Source: CAD feature listing. Evaluate the final solid. Frame: model axes, mm. A direction names the side the tool comes from. Give positions to 0.01 mm unless a question says otherwise; leave off trailing zeros. Write each loop counter-clockwise with the first axis right and the second up, starting at its lowest first coordinate (ties: lowest second). Pieces come first, ordered by that corner, then holes. Notation, with made-up numbers: (3.5, 86) -> (11.5, 86) arc R17 ccw to (11.5, 91) -> close; hole circle Ø7 at (-0.5, 46.25). An arc over 180 degrees is marked (long way). Use one line per item in the form item = value. Start each with the question number.
(1) Cut plane C-C, the plane z = 6.5. Count the separate pieces of the cut face and the enclosed holes in it, and give its area (3 significant figures).
(2) Material intervals for line 1 along Y through (x, z) = (13, 47); line 2 along Y through (x, z) = (-0.5, 20); line 3 along Y through (x, z) = (57, 85), sorted ascending. Write a range as from..to.
(3) Set-up query: faces 1 (the face through (55.105, 11.711, 44.37)), 2 (the face through (61.38, 10.58, 92.99)), 3 (the face through (-6.07, 42.42, 92.99)), 4 (the face through (62.657, 26, 52)). Return all of +Z, -Z, +X, -X, +Y, -Y with unobstructed straight access to the full face (end or side cutting, diameter ignored); none if empty.
(4) Cut plane A-A, the plane y = 29. Output: boundary loops of the cut face in (x, z).
(5) Draft query along X for faces 5 (the face through (55.18, 41.38, 44.37)), 6 (the face through (-6.135, 44.919, 93.208)), 7 (the face through (27, 0, 47)). Return one class per face: pulls with the +X half, pulls with the -X half, needs draft (parallel to the pull), parting line crosses it, or undercut.
(6) Cut plane B-B, the plane x = 16.5. Output: boundary loops of the cut face in (y, z).
(7) First-contact query: P1, Ø0.7, axis at x = 60.5, z = 51, coming from the -Y side; P2, Ø5, axis at x = 59.76, y = 37.5, coming from the +Z side; P3, Ø2, axis at x = 31, y = 43, coming from the -Z side. Flat tips, straight axial feed; report the tip coordinate or a pass-through.
from build123d import *

# Parameters (mm, degrees)
BOSS_EXTRUDE1_DEPTH = 90
SKETCH1_3_R         = 2.125
BOSS_EXTRUDE2_DEPTH = 10
FILLET1_R           = 2
BOSS_EXTRUDE3_START = 4
BOSS_EXTRUDE3_DEPTH = 4
CHAMFER1_SIZE       = 2
FILLET3_R           = 3


with BuildPart() as part:
    # Sketch1 → Boss-Extrude1 (new body)
    with BuildSketch(Plane.XY):
        with BuildLine():
            Line((55.313708499, 53), (0, 53))
            Line((0, 53), (-7.343145751, 45.656854249))
            Line((-7.343145751, 45.656854249), (-7.343145751, 41.125))
            Line((-7.343145751, 41.125), (-4.443145751, 41.125))
            ThreePointArc((-4.443145751, 41.125), (-0.818145751, 37.5), (-4.443145751, 33.875))
            Line((-4.443145751, 33.875), (-7.343145751, 33.875))
            Line((-7.343145751, 33.875), (-7.343145751, 19.125))
            Line((-7.343145751, 19.125), (-4.443145751, 19.125))
            ThreePointArc((-4.443145751, 19.125), (-0.818145751, 15.5), (-4.443145751, 11.875))
            Line((-4.443145751, 11.875), (-7.343145751, 11.875))
            Line((-7.343145751, 11.875), (-7.343145751, 7.343145751))
            Line((-7.343145751, 7.343145751), (0, 0))
            Line((0, 0), (55.313708499, 0))
            Line((55.313708499, 0), (62.656854249, 7.343145751))
            Line((62.656854249, 7.343145751), (62.656854249, 11.875))
            Line((62.656854249, 11.875), (59.756854249, 11.875))
            ThreePointArc((59.756854249, 11.875), (56.131854249, 15.5), (59.756854249, 19.125))
            Line((59.756854249, 19.125), (62.656854249, 19.125))
            Line((62.656854249, 19.125), (62.656854249, 33.875))
            Line((62.656854249, 33.875), (59.756854249, 33.875))
            ThreePointArc((59.756854249, 33.875), (56.131854249, 37.5), (59.756854249, 41.125))
            Line((59.756854249, 41.125), (62.656854249, 41.125))
            Line((62.656854249, 41.125), (62.656854249, 45.656854249))
            Line((62.656854249, 45.656854249), (55.313708499, 53))
        make_face()
        with BuildLine():
            Line((53.656854249, 4), (1.656854249, 4))
            Line((1.656854249, 4), (-3.343145751, 9))
            Line((-3.343145751, 9), (-3.343145751, 9.601695159))
            ThreePointArc((-3.343145751, 9.601695159), (0.172046553, 11.665942097), (1.556854249, 15.5))
            Line((1.556854249, 15.5), (1.556854249, 37.5))
            ThreePointArc((1.556854249, 37.5), (0.172046553, 41.334057903), (-3.343145751, 43.398304841))
            Line((-3.343145751, 43.398304841), (-3.343145751, 44))
            Line((-3.343145751, 44), (1.656854249, 49))
            Line((1.656854249, 49), (53.656854249, 49))
            Line((53.656854249, 49), (58.656854249, 44))
            Line((58.656854249, 44), (58.656854249, 43.398304841))
            ThreePointArc((58.656854249, 43.398304841), (55.141661946, 41.334057903), (53.756854249, 37.5))
            Line((53.756854249, 37.5), (53.756854249, 15.5))
            ThreePointArc((53.756854249, 15.5), (55.141661946, 11.665942097), (58.656854249, 9.601695159))
            Line((58.656854249, 9.601695159), (58.656854249, 9))
            Line((58.656854249, 9), (53.656854249, 4))
        make_face(mode=Mode.SUBTRACT)
    extrude(amount=BOSS_EXTRUDE1_DEPTH)

    # Sketch1<3> → Boss-Extrude2 (add)
    # profile 1 of 2: a face of its own
    with BuildSketch(Plane.XY):
        with BuildLine():
            ThreePointArc((-4.443145751, 33.875), (-0.818145751, 37.5), (-4.443145751, 41.125))
            Line((-4.443145751, 41.125), (-7.343145751, 41.125))
            Line((-7.343145751, 41.125), (-7.343145751, 44.1))
            Line((-7.343145751, 44.1), (-9.943145751, 41.5))
            Line((-9.943145751, 41.5), (-9.943145751, 11.5))
            Line((-9.943145751, 11.5), (-7.343145751, 8.9))
            Line((-7.343145751, 8.9), (-7.343145751, 11.875))
            Line((-7.343145751, 11.875), (-4.443145751, 11.875))
            ThreePointArc((-4.443145751, 11.875), (-0.818145751, 15.5), (-4.443145751, 19.125))
            Line((-4.443145751, 19.125), (-7.343145751, 19.125))
            Line((-7.343145751, 19.125), (-7.343145751, 33.875))
            Line((-7.343145751, 33.875), (-4.443145751, 33.875))
        make_face()
        with Locations((-4.443145751, 15.5)):
            Circle(SKETCH1_3_R, mode=Mode.SUBTRACT)
        with Locations((-4.443145751, 37.5)):
            Circle(SKETCH1_3_R, mode=Mode.SUBTRACT)
    # profile 2 of 2: a face of its own
    with BuildSketch(Plane.XY):
        with BuildLine():
            Line((65.256854249, 41.5), (62.656854249, 44.1))
            Line((62.656854249, 44.1), (62.656854249, 41.125))
            Line((62.656854249, 41.125), (59.756854249, 41.125))
            ThreePointArc((59.756854249, 41.125), (56.131854249, 37.5), (59.756854249, 33.875))
            Line((59.756854249, 33.875), (62.656854249, 33.875))
            Line((62.656854249, 33.875), (62.656854249, 19.125))
            Line((62.656854249, 19.125), (59.756854249, 19.125))
            ThreePointArc((59.756854249, 19.125), (56.131854249, 15.5), (59.756854249, 11.875))
            Line((59.756854249, 11.875), (62.656854249, 11.875))
            Line((62.656854249, 11.875), (62.656854249, 8.9))
            Line((62.656854249, 8.9), (65.256854249, 11.5))
            Line((65.256854249, 11.5), (65.256854249, 41.5))
        make_face()
        with Locations((59.756854249, 37.5)):
            Circle(SKETCH1_3_R, mode=Mode.SUBTRACT)
        with Locations((59.756854249, 15.5)):
            Circle(SKETCH1_3_R, mode=Mode.SUBTRACT)
    extrude(amount=BOSS_EXTRUDE2_DEPTH)

    # Fillet1
    fillet1_edges = [part.edges().sort_by_distance(p)[0] for p in [
        (62.656854249, 41.125, 50),
        (62.656854249, 33.875, 50),
        (62.656854249, 19.125, 50),
        (62.656854249, 11.875, 50),
        (-7.343145751, 11.875, 50),
        (-7.343145751, 19.125, 50),
        (-7.343145751, 33.875, 50),
        (-7.343145751, 41.125, 50),
    ]]
    fillet(fillet1_edges, radius=FILLET1_R)

    # Sketch2 → Boss-Extrude3 (add)
    with BuildSketch(Plane.XY.offset(90).offset(BOSS_EXTRUDE3_START)):
        with BuildLine():
            Line((-7.343145751, 31.875), (-7.343145751, 21.125))
            ThreePointArc((-7.343145751, 21.125), (-6.757359313, 19.710786438), (-5.343145751, 19.125))
            Line((-5.343145751, 19.125), (-4.443145751, 19.125))
            ThreePointArc((-4.443145751, 19.125), (-0.818145751, 15.5), (-4.443145751, 11.875))
            Line((-4.443145751, 11.875), (-5.343145751, 11.875))
            ThreePointArc((-5.343145751, 11.875), (-6.757359313, 11.289213562), (-7.343145751, 9.875))
            Line((-7.343145751, 9.875), (-7.343145751, 7.343145751))
            Line((-7.343145751, 7.343145751), (0, 0))
            Line((0, 0), (55.313708499, 0))
            Line((55.313708499, 0), (62.656854249, 7.343145751))
            Line((62.656854249, 7.343145751), (62.656854249, 9.875))
            ThreePointArc((62.656854249, 9.875), (62.071067812, 11.289213562), (60.656854249, 11.875))
            Line((60.656854249, 11.875), (59.756854249, 11.875))
            ThreePointArc((59.756854249, 11.875), (56.131854249, 15.5), (59.756854249, 19.125))
            Line((59.756854249, 19.125), (60.656854249, 19.125))
            ThreePointArc((60.656854249, 19.125), (62.071067812, 19.710786438), (62.656854249, 21.125))
            Line((62.656854249, 21.125), (62.656854249, 31.875))
            ThreePointArc((62.656854249, 31.875), (62.071067812, 33.289213562), (60.656854249, 33.875))
            Line((60.656854249, 33.875), (59.756854249, 33.875))
            ThreePointArc((59.756854249, 33.875), (56.131854249, 37.5), (59.756854249, 41.125))
            Line((59.756854249, 41.125), (60.656854249, 41.125))
            ThreePointArc((60.656854249, 41.125), (62.071067812, 41.710786438), (62.656854249, 43.125))
            Line((62.656854249, 43.125), (62.656854249, 45.656854249))
            Line((62.656854249, 45.656854249), (55.313708499, 53))
            Line((55.313708499, 53), (0, 53))
            Line((0, 53), (-7.343145751, 45.656854249))
            Line((-7.343145751, 45.656854249), (-7.343145751, 43.125))
            ThreePointArc((-7.343145751, 43.125), (-6.757359313, 41.710786438), (-5.343145751, 41.125))
            Line((-5.343145751, 41.125), (-4.443145751, 41.125))
            ThreePointArc((-4.443145751, 41.125), (-0.818145751, 37.5), (-4.443145751, 33.875))
            Line((-4.443145751, 33.875), (-5.343145751, 33.875))
            ThreePointArc((-5.343145751, 33.875), (-6.757359313, 33.289213562), (-7.343145751, 31.875))
        make_face()
    extrude(amount=-BOSS_EXTRUDE3_DEPTH)

    # Chamfer1
    chamfer1_edges = [part.edges().sort_by_distance(p)[0] for p in [
        (-7.343145751, 44.390927125, 94),
        (-6.757359313, 41.710786438, 94),
        (-4.893145751, 41.125, 94),
        (-0.818145751, 37.5, 94),
        (-4.893145751, 33.875, 94),
        (-6.757359313, 33.289213562, 94),
        (-7.343145751, 26.5, 94),
        (-6.757359313, 19.710786438, 94),
        (-4.893145751, 19.125, 94),
        (-0.818145751, 15.5, 94),
        (-4.893145751, 11.875, 94),
        (-6.757359313, 11.289213562, 94),
        (-7.343145751, 8.609072875, 94),
        (27.656854249, 0, 94),
        (62.656854249, 8.609072875, 94),
        (62.071067812, 11.289213562, 94),
        (60.206854249, 11.875, 94),
        (56.131854249, 15.5, 94),
        (60.206854249, 19.125, 94),
        (62.071067812, 19.710786438, 94),
        (62.656854249, 26.5, 94),
        (62.071067812, 33.289213562, 94),
        (60.206854249, 33.875, 94),
        (56.131854249, 37.5, 94),
        (60.206854249, 41.125, 94),
        (62.071067812, 41.710786438, 94),
        (62.656854249, 44.390927125, 94),
        (27.656854249, 53, 94),
    ]]
    chamfer(chamfer1_edges, length=CHAMFER1_SIZE - 0.0001)  # a hair under: the kernel refuses the full size

    # Fillet3
    fillet3_edges = [part.edges().sort_by_distance(p)[0] for p in [
        (-9.943145751, 41.5, 5),
        (-9.943145751, 11.5, 5),
        (65.256854249, 11.5, 5),
        (65.256854249, 41.5, 5),
        (62.656854249, 7.343145751, 46.00005),
        (55.313708499, 0, 46.00005),
        (0, 0, 46.00005),
        (-7.343145751, 7.343145751, 46.00005),
        (55.313708499, 53, 46.00005),
        (62.656854249, 45.656854249, 46.00005),
        (-7.343145751, 45.656854249, 46.00005),
        (0, 53, 46.00005),
    ]]
    fillet(fillet3_edges, radius=FILLET3_R)


solid = part.part
Geometry says:
q1.separate_pieces = 1
q1.enclosed_holes = 5
q1.area = 1,280 mm^2
q2.line_1 = 0..4, 49..53
q2.line_2 = 0.56..6.16, 10.98..42.02, 46.84..52.44
q2.line_3 = 1.69..7.34, 10.17..13.15, 17.85..35.15, 39.85..42.83, 45.66..51.31
q3.face_1 = -Z
q3.face_2 = +Z, +X
q3.face_3 = +Z, -X
q3.face_4 = +Z, +X, +Y, -Y
q4.outline = (-9.94, 0) -> (1.56, 0) -> (1.56, 90) -> (53.76, 90) -> (53.76, 0) -> (65.26, 0) -> (65.26, 10) -> (62.66, 10) -> (62.66, 92) -> (60.66, 94) -> (-5.34, 94) -> (-7.34, 92) -> (-7.34, 10) -> (-9.94, 10) -> close
q5.face_5 = undercut
q5.face_6 = pulls with the -X half
q5.face_7 = needs draft
q6.outline = (0, 0) -> (4, 0) -> (4, 90) -> (49, 90) -> (49, 0) -> (53, 0) -> (53, 92) -> (51, 94) -> (2, 94) -> (0, 92) -> close
q7.P1 = 4.84
q7.P2 = 10
q7.P3 = 90
